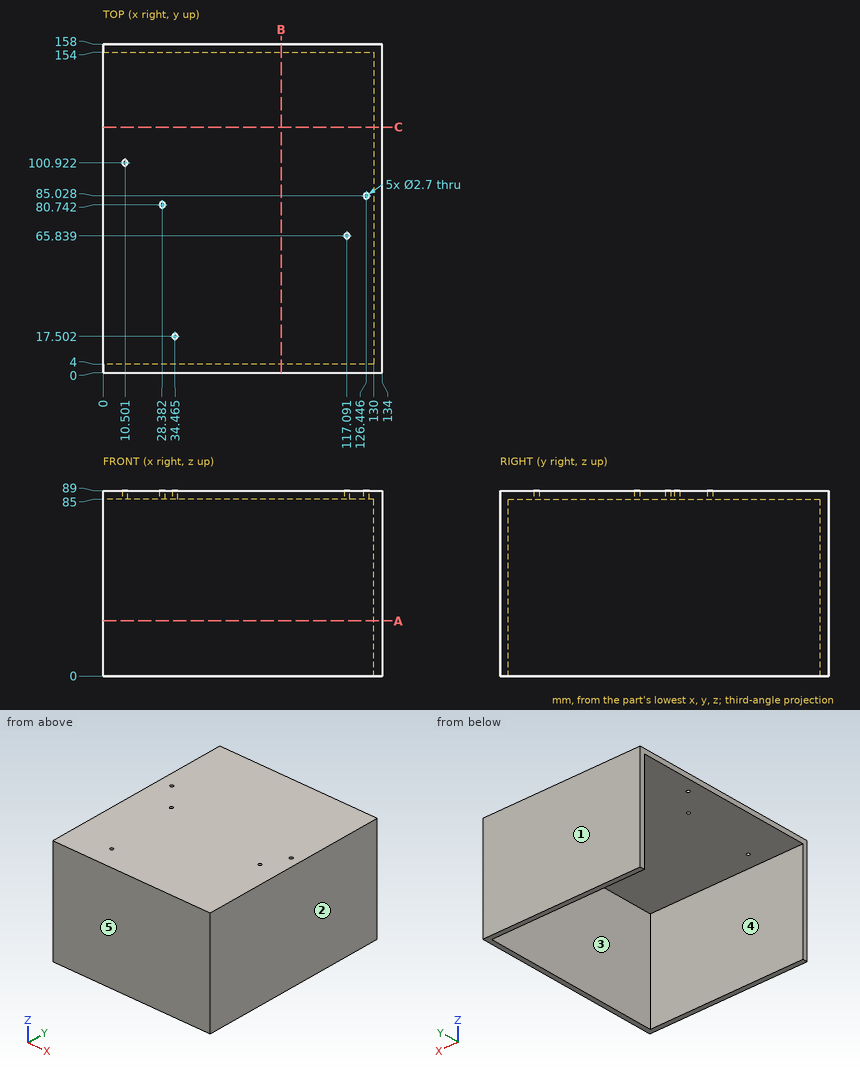
Design review of the part shown in the three views and the two pictorial views. Dimensions are in mm from the part's minimum x, y and z. A direction names the side the tool comes from. Round coordinates to 2 decimals unless told otherwise and drop trailing zeros. Loops run counter-clockwise (first coordinate to the right, second up) from the corner with the lowest first, then second, coordinate; pieces in that order, holes last. Notation, with made-up numbers: (-37, 60.5) -> (-7, 60.5) arc R10 ccw to (-7, 65.5) -> close; hole circle Ø3 at (69, 46.25). An arc over 180 degrees is marked (long way). Return JSON: item names as keys, results as strings.
(1) For the marked faces 4 and 5, list the 3-axis set-ups (+Z, -Z, +X, -X, +Y, -Y) from which the entire face can be reached by the end or side of a thin tool; tool diameter is ignored.
Solved:
{"face 4": "-Z, -X", "face 5": "+Z, -Z, +X, -X, -Y"}
(2) Add section A-A on z = 26.5. Write out the cut boundary in (x, y), plus the area to 3 significant figures.
Solved:
{"outline": "(0, 0) -> (134, 0) -> (134, 158) -> (0, 158) -> (0, 154) -> (130, 154) -> (130, 4) -> (0, 4) -> close", "area": "1,670 mm2"}
(3) The part is to be moulded in two halves that separate along Y. For the marked faces 1, 2 and 3, say which applies: released by +Y, released by -Y, zero draft, split by the parting line, or undercut.
Solved:
{"face 1": "released by +Y", "face 2": "zero draft", "face 3": "undercut"}
(4) For pin 1 (5 mm diameter, centred on y = 140.5, z = 32.5, fed in from -X); pin 2 (4.5 mm diameter, centred on x = 28.38, y = 80.74, fed in from -Z), all flat-tipped, find the tip position at first contact; note any pin that passes through.
Solved:
{"pin 1": "x = 130", "pin 2": "z = 85"}
(5) Add section C-C on y = 118. Write out the cut boundary in (x, z), plus the area to 3 significant figures.
Solved:
{"outline": "(0, 85) -> (130, 85) -> (130, 0) -> (134, 0) -> (134, 89) -> (0, 89) -> close", "area": "876 mm2"}
(6) For line 1 (Y direction, x = 90, z = 74.5); line 2 (Z direction, x = 110.5, y = 91); line 3 (X direction, y = 40.5, z = 35), list the stretches that pass through material, from the lowest coordinate up.
Solved:
{"line 1": "0 to 4, 154 to 158", "line 2": "85 to 89", "line 3": "130 to 134"}
(7) Add section B-B on x = 85.5. Write out the cut boundary in (y, z).
Solved:
{"outline": "(0, 0) -> (4, 0) -> (4, 85) -> (154, 85) -> (154, 0) -> (158, 0) -> (158, 89) -> (0, 89) -> close"}
